```python
from build123d import *

# Parameters (mm, degrees)
SKETCH1_W                 = 17.78
SKETCH1_H                 = 17.78
SKETCH1_R                 = 4.7625
BOSS_EXTRUDE1_DEPTH       = 6.35
F_8_32_TAPPED_HOLE1_D     = 3.4544
F_8_32_TAPPED_HOLE1_DEPTH = 9.630193539
F_8_32_TAPPED_HOLE1_TIP   = 1.037806461


with BuildPart() as part:
    # Sketch1 → Boss-Extrude1 (new body)
    with BuildSketch(Plane(origin=(0, 0, 0), x_dir=(1, 0, 0), z_dir=(0, 1, 0))):
        Rectangle(SKETCH1_W, SKETCH1_H)
        with Locations(Location((0, 0, 0), (0, 0, 270))):
            Circle(SKETCH1_R, mode=Mode.SUBTRACT)
    extrude(amount=BOSS_EXTRUDE1_DEPTH)

    # #8-32 Tapped Hole1
    with Locations(Plane.XY.offset(8.89)):
        with Locations((0, 3.175)):
            Hole(F_8_32_TAPPED_HOLE1_D / 2, depth=F_8_32_TAPPED_HOLE1_DEPTH)
            with Locations((0, 0, -(F_8_32_TAPPED_HOLE1_DEPTH + F_8_32_TAPPED_HOLE1_TIP / 2))):  # 118° drill point
                Cone(0, F_8_32_TAPPED_HOLE1_D / 2, F_8_32_TAPPED_HOLE1_TIP, mode=Mode.SUBTRACT)

    # Sketch7 → #8-32 Tapped Hole2 (revolve, cut)
    with BuildSketch(Plane(origin=(-8.89, 3.175, 3.175), x_dir=(0, 0, 1), z_dir=(0, 1, 0))):
        Polygon((0, 0), (0, 4.847806461), (1.7272, 3.81), (1.7272, 0), align=None)
    f_8_32_tapped_hole2 = revolve(axis=Axis((-15.24, 3.175, 3.175), (1, 0, 0)), mode=Mode.SUBTRACT)

    # Mirror1: #8-32 Tapped Hole2 across plane
    add(f_8_32_tapped_hole2.mirror(Plane(origin=(0, 0, 0), x_dir=(0, 0, 1), z_dir=(1, 0, 0))), mode=Mode.SUBTRACT)


solid = part.part
```
Work out the finished part from the listing and answer in its coordinate system (mm). A direction names the side the tool comes from. Round coordinates to 2 decimals unless told otherwise and drop trailing zeros. Loops run counter-clockwise (first coordinate to the right, second up) from the corner with the lowest first, then second, coordinate; pieces in that order, holes last. Notation, with made-up numbers: (16, 87) -> (32, 87) arc R24 cw to (32, 101) -> close; hole circle Ø2 at (33, 84.25). An arc over 180 degrees is marked (long way). Write each question's results on one line, items separated by ' | '. Start each with the question number.
1. A tool of negligible diameter and unlimited length cuts with its end or side. For faces 1 (the face through (4, 6.35, -4)), 2 (the face through (1.726, 3.251, 6.633)), 3 (the face through (-7.012, 4.226, 1.804)), from which of +Z, -Z, +X, -X, +Y, -Y can it reach the whole face along a straight path? Write none if from no direction.
2. Find the intervals of material crossed by probe 1 along X at (y, z) = (1.5, 0); probe 2 along X at (y, z) = (3.75, -4); probe 3 along Z at (x, y) = (-6.75, 2), in increasing order. Write a range as from..to.
3. Given pin 1 Ø1 at (x, z) = (0.5, 5.5) entering from -Y; pin 2 Ø2 at (y, z) = (3.175, 3.175) entering from -X; pin 3 Ø3 at (x, y) = (0, 3.175) entering from +Z, each flat-ended and moving along its own axis, determine where each tip first touches the part or whether it passes through.
4. Section A-A (x = 0) is taken. Determine the outline of the cut face in (y, z), plus the area to 3 significant figures.
5. Section C-C (x = 6) is taken. Determine the outline of the cut face in (y, z) (3 decimals), plus the area to 3 significant figures.
6. For a pull along Z with two mould halves and no side action, classify faces 4 (the face through (2, 3, 8.89)), 5 (the face through (7.012, 4.226, 1.804)), 6 (the face through (8.89, 3, 0)) as +Z half, -Z half, draft (parallel to the pull), parting line (faces both ways), or undercut.
7. Section B-B (z = 0) is taken. Determine the outline of the cut face in (x, y).
8. Section D-D (x = 3) is taken. Determine the outline of the cut face in (y, z).
Evaluation:
1) face 1: +Z, -Z, +X, -X, +Y | face 2: +Z | face 3: -X
2) probe 1: x = -8.89..-4.76, 4.76..8.89 | probe 2: x = -8.89..-2.58, 2.58..8.89 | probe 3: z = -8.89..1.91, 4.44..8.89
3) pin 1: stops at y = 0 | pin 2: stops at x = -4.64 | pin 3: stops at z = -4.52
4) outline: (0, -8.89) -> (6.35, -8.89) -> (6.35, -4.76) -> (0, -4.76) -> close; (0, 4.76) -> (1.45, 4.76) -> (1.45, 8.89) -> (0, 8.89) -> close; (4.9, 4.76) -> (6.35, 4.76) -> (6.35, 8.89) -> (4.9, 8.89) -> close | area: 38.2 mm2
5) outline: (0, -8.89) -> (6.35, -8.89) -> (6.35, 8.89) -> (0, 8.89) -> close; hole circle Ø3.454 at (3.175, 3.175) | area: 104 mm2
6) face 4: +Z half | face 5: undercut | face 6: draft
7) outline: (-8.89, 0) -> (-4.76, 0) -> (-4.76, 6.35) -> (-8.89, 6.35) -> close; (4.76, 0) -> (8.89, 0) -> (8.89, 6.35) -> (4.76, 6.35) -> close
8) outline: (0, -8.89) -> (6.35, -8.89) -> (6.35, -3.7) -> (0, -3.7) -> close; (0, 3.7) -> (6.35, 3.7) -> (6.35, 8.89) -> (0, 8.89) -> close
